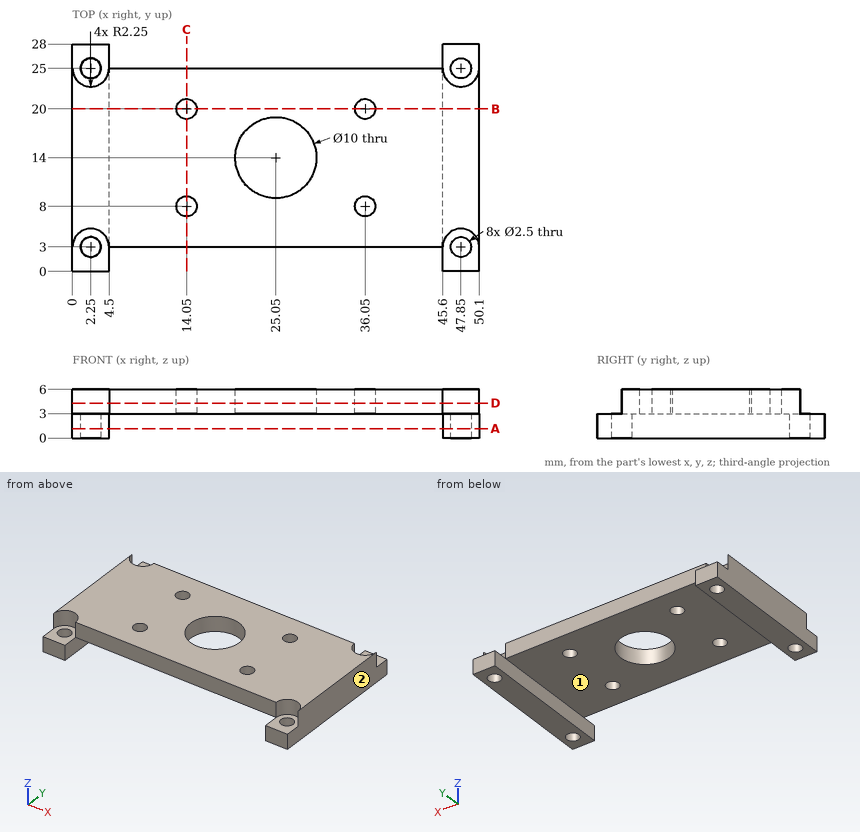
Geometry: see drawing. Coordinates: mm, zero at the bounding-box minimum. A direction names the side the tool comes from. Give positions to 0.01 mm unless a question says otherwise; leave off trailing zeros. Write each loop counter-clockwise with the first axis right and the second up, starting at its lowest first coordinate (ties: lowest second). Pieces come first, ordered by that corner, then holes. Notation, with made-up numbers: (-34, -8.75) - (9, -8.75) arc R18 ccw to (9, 0.25) - close; hole circle Ø10 at (1, -10). An arc over 180 degrees is marked (long way). Return JSON: item names as keys, results as strings. Group by question number.
1) Set-up query: the marked faces 1 and 2. Return all of +Z, -Z, +X, -X, +Y, -Y with unobstructed straight access to the full face (end or side cutting, diameter ignored); none if empty.
2) Section A-A on z = 1.15. Return the cut outline in (x, y), plus the area to 3 significant figures.
3) Section C-C on x = 14.05. Return the cut outline in (y, z), plus the area to 3 significant figures.
4) Section D-D on z = 4.3. Return the cut outline in (x, y).
5) First-contact query: P1, Ø2, axis at x = 14.05, y = 20, coming from the +Z side; P2, Ø3, axis at x = 36.05, y = 8, coming from the -Z side; P3, Ø3.5, axis at x = 2, y = 25, coming from the +Z side; P4, Ø3.5, axis at x = 20.5, z = 4, coming from the -Y side. Flat tips, straight axial feed; report the tip coordinate or a pass-through.
6) Section B-B on y = 20. Return the cut outline in (x, z).
7) Line query: line 1 (Y direction, x = 14.05, z = 4.35); line 2 (X direction, y = 20, z = 1.25); line 3 (X direction, y = 4, z = 4.95). Output: solid intervals per line, ascending.
Filled in:
{
 "1": {"face 1": "-Z, +Y, -Y", "face 2": "+Z, -Z, +X, +Y, -Y"},
 "2": {"outline": "(0, 0) - (4.5, 0) - (4.5, 28) - (0, 28) - close; (45.6, 0) - (50.1, 0) - (50.1, 28) - (45.6, 28) - close; hole circle Ø2.5 at (2.25, 3); hole circle Ø2.5 at (2.25, 25); hole circle Ø2.5 at (47.85, 3); hole circle Ø2.5 at (47.85, 25)", "area": "232 mm^2"},
 "3": {"outline": "(3, 3) - (6.75, 3) - (6.75, 6) - (3, 6) - close; (9.25, 3) - (18.75, 3) - (18.75, 6) - (9.25, 6) - close; (21.25, 3) - (25, 3) - (25, 6) - (21.25, 6) - close", "area": "51.0 mm^2"},
 "4": {"outline": "(0, 3) arc R2.25 cw to (4.5, 3) - (45.6, 3) arc R2.25 cw to (50.1, 3) - (50.1, 25) arc R2.25 cw to (45.6, 25) - (4.5, 25) arc R2.25 cw to (0, 25) - close; hole circle Ø2.5 at (14.05, 8); hole circle Ø2.5 at (14.05, 20); hole circle Ø10 at (25.05, 14); hole circle Ø2.5 at (36.05, 8); hole circle Ø2.5 at (36.05, 20)"},
 "5": {"P1": "passes through", "P2": "stops at z = 3", "P3": "stops at z = 3", "P4": "stops at y = 3"},
 "6": {"outline": "(0, 0) - (4.5, 0) - (4.5, 3) - (12.8, 3) - (12.8, 6) - (0, 6) - close; (15.3, 3) - (34.8, 3) - (34.8, 6) - (15.3, 6) - close; (37.3, 3) - (45.6, 3) - (45.6, 0) - (50.1, 0) - (50.1, 6) - (37.3, 6) - close"},
 "7": {"line 1": "y = 3 to 6.75, 9.25 to 18.75, 21.25 to 25", "line 2": "x = 0 to 4.5, 45.6 to 50.1", "line 3": "x = 0 to 0.23, 4.27 to 45.83, 49.87 to 50.1"}
}
